from build123d import *

# Parameters (mm, degrees)
BOSS_EXTRUDE1_DEPTH = 2.7


with BuildPart() as part:
    # Sketch1 → Boss-Extrude1 (new body)
    with BuildSketch(Plane.XY):
        Polygon((80, -17.5), (82.7, -17.5), (82.7, -27.5), (80, -27.5), (80, -37.5), (82.7, -37.5), (82.7, -47.5), (80, -47.5), (-80, -47.5), (-82.7, -47.5), (-82.7, -37.5), (-80, -37.5), (-80, -27.5), (-82.7, -27.5), (-82.7, -17.5), (-80, -17.5), (-80, -7.5), (-82.7, -7.5), (-82.7, 2.5), (-80, 2.5), (-80, 12.5), (-82.7, 12.5), (-82.7, 22.5), (-80, 22.5), (-80, 32.5), (-82.7, 32.5), (-82.7, 42.5), (-80, 42.5), (-80, 47.5), (80, 47.5), (80, 42.5), (82.7, 42.5), (82.7, 32.5), (80, 32.5), (80, 22.5), (82.7, 22.5), (82.7, 12.5), (80, 12.5), (80, 2.5), (82.7, 2.5), (82.7, -7.5), (80, -7.5), align=None)
        with BuildLine():
            ThreePointArc((-7.5, 6.614378278), (0, -10), (7.5, 6.614378278))
            Line((7.5, 6.614378278), (-7.5, 6.614378278))
        make_face(mode=Mode.SUBTRACT)
    extrude(amount=BOSS_EXTRUDE1_DEPTH)


solid = part.part
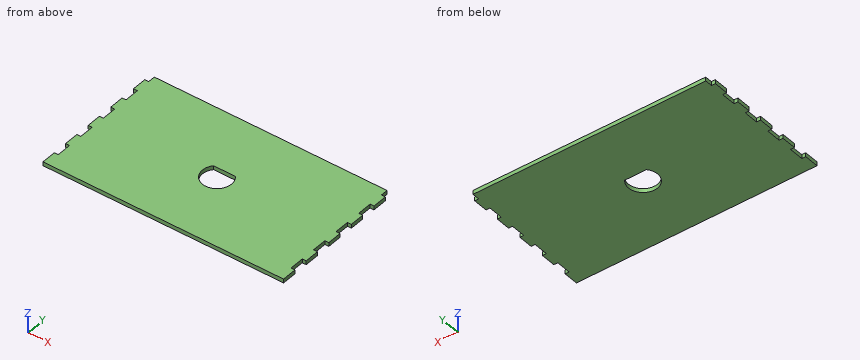
Work out the finished part from the listing and answer in its coordinate system (mm). Round coordinates to 2 decimals unless told otherwise and drop trailing zeros. Order: outer loops, then holes, each group sorted by start corner. A loop starts at its lowest first (then second) coordinate and runs counter-clockwise, first axis right, second up. Notation, with made-up numbers: M 71.5,49 L 79.5,49 A14 ccw 79.5,68 Z; hole C -27,-16.75 d2. An arc over 180 degrees is marked long. Put each result on its own line as item: value. Start each with the question number.
Q1. Section C-C, the plane y = 28 is taken. Write down the section's boundary in (x, z).
Q2. Flat-ended cylindrical pins translate along their axes: pin 1 (0.8 mm diameter, centred on y = 5.5, z = 1.5, fed in from +X); pin 2 (1.4 mm diameter, centred on y = -13.5, z = 1, fed in from -X); pin 3 (0.8 mm diameter, centred on x = -81, z = 1.5, fed in from +Y). Find the tip coordinate at first contact, or state that the pin passes through.
Q3. Section B-B, the plane y = 0 is taken. Write down the section's boundary in (x, z).
Q4. Section A-A, the plane x = 0 is taken. Write down the section's boundary in (y, z), and give its area (3 significant figures).
Q5. Straight lines are drawn through the part: L1, parallel to X at y = 0, z = 1.4; L2, parallel to Y at x = 0, z = 1.1; L3, parallel to X at y = 9, z = 0.65. For each, find the intervals that lie inside material, in ascending order. Write a range as [from, to].
Findings below:
1. outline: M -80,0 L 80,0 L 80,2.7 L -80,2.7 Z
2. pin 1: stops at x = 80
2. pin 2: stops at x = -80
2. pin 3: stops at y = 42.5
3. outline: M -82.7,0 L -10,0 L -10,2.7 L -82.7,2.7 Z; M 10,0 L 82.7,0 L 82.7,2.7 L 10,2.7 Z
4. outline: M -47.5,0 L -10,0 L -10,2.7 L -47.5,2.7 Z; M 6.61,0 L 47.5,0 L 47.5,2.7 L 6.61,2.7 Z
4. area: 212 mm^2
5. L1: x = [-82.7, -10], [10, 82.7]
5. L2: y = [-47.5, -10], [6.61, 47.5]
5. L3: x = [-80, 80]
